```python
from build123d import *

# Parameters (mm, degrees)
SZKIC1_R                    = 40
DODANIE_WYCI_GNI_CIE1_DEPTH = 250
SZKIC2_W                    = 120
SZKIC2_H                    = 80
DODANIE_WYCI_GNI_CIE2_DEPTH = 10
SZKIC3_W                    = 10
SZKIC3_H                    = 80
DODANIE_WYCI_GNI_CIE3_DEPTH = 50


with BuildPart() as part:
    # Szkic1 → Dodanie-wyciągnięcie1 (new body)
    with BuildSketch(Plane.XY):
        Circle(SZKIC1_R)
    extrude(amount=DODANIE_WYCI_GNI_CIE1_DEPTH)

    # Szkic2 → Dodanie-wyciągnięcie2 (add)
    with BuildSketch(Plane.XY.offset(250)):
        Rectangle(SZKIC2_W, SZKIC2_H)
    extrude(amount=DODANIE_WYCI_GNI_CIE2_DEPTH)

    # Szkic3 → Dodanie-wyciągnięcie3 (add)
    with BuildSketch(Plane.XY.offset(260)):
        with Locations((-55, 0)):
            Rectangle(SZKIC3_W, SZKIC3_H)
        with Locations((55, 0)):
            Rectangle(SZKIC3_W, SZKIC3_H)
    extrude(amount=DODANIE_WYCI_GNI_CIE3_DEPTH)


solid = part.part
```
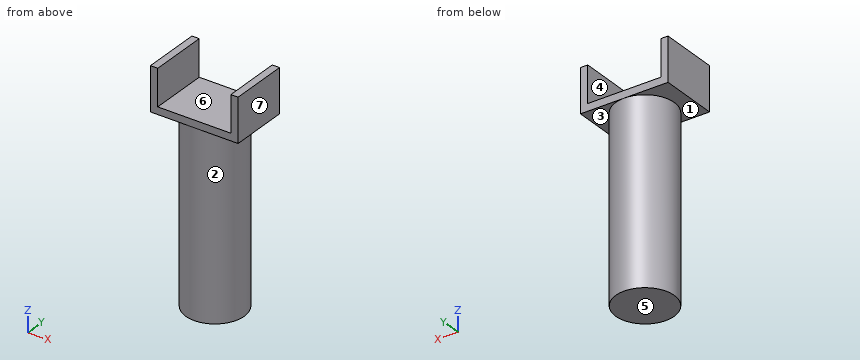
The model under review builds one solid part; all positions refer to its coordinate system, in mm. Face numbers are marked on the shaded views. A direction names the side the tool comes from. Round coordinates to 2 decimals unless told otherwise and drop trailing zeros. Loops run counter-clockwise (first coordinate to the right, second up) from the corner with the lowest first, then second, coordinate; pieces in that order, holes last. Notation, with made-up numbers: M 14.5,65.25 L 30.5,65.25 A12 cw 30.5,73.25 Z; hole C -3.75,48 d2. An arc over 180 degrees is marked long. Put each result on its own line as item: value.
Q1. Consider section C-C, the plane x = 34. Give the boundary of the cut face in (y, z).
Result set:
outline: M -40,250 L -21.07,250 L -21.07,0 L 21.07,0 L 21.07,250 L 40,250 L 40,260 L -40,260 Z
Q2. Consider section A-A, the plane z = 288.5. Give the boundary of the cut face in (x, y).
Result set:
outline: M -60,-40 L -50,-40 L -50,40 L -60,40 Z; M 50,-40 L 60,-40 L 60,40 L 50,40 Z
Q3. Consider section D-D, the plane z = 34. Give the boundary of the cut face in (x, y), then the cut area to 3 significant figures.
Result set:
outline: C 0,0 d80
area: 5,030 mm²
Q4. Consider section B-B, the plane y = 0. Give the boundary of the cut face in (x, z), then the cut area to 3 significant figures.
Result set:
outline: M -60,250 L -40,250 L -40,0 L 40,0 L 40,250 L 60,250 L 60,310 L 50,310 L 50,260 L -50,260 L -50,310 L -60,310 Z
area: 22,200 mm²
Q5. For pin 1 (4 mm diameter, centred on x = -6.5, z = 208.5, fed in from -Y); pin 2 (8 mm diameter, centred on y = 14.5, z = 73.5, fed in from -X); pin 3 (4 mm diameter, centred on x = 41.5, y = 10, fed in from -Z), all flat-tipped, find the tip position at first contact; note any pin that passes through.
Result set:
pin 1: stops at y = -39.75
pin 2: stops at x = -38.6
pin 3: stops at z = 250
Q6. To check wall thickness, follow L1, parallel to X at y = 20.5, z = 280.5; L2, parallel to Z at x = 23.5, y = 36; L3, parallel to Z at x = 23, y = 32. State the ranges of each line that lie inside material, in increasing order.
Result set:
L1: x = -60 to -50, 50 to 60
L2: z = 250 to 260
L3: z = 0 to 260
Q7. Machinability: for the marked faces 1, 2, 3 and 4, which of the approach directions +Z, -Z, +X, -X, +Y, -Y give a long, thin tool a straight path to every point of the face, cutting with its end or side? Answer none if there is none.
Result set:
face 1: -Z, -X
face 2: -Z
face 3: -Z, +X
face 4: +Z, +Y, -Y
Q8. Mouldability with a two-part tool opening along X and no side actions: class the marked faces 5, 6 and 7 as released by +X, released by -X, zero draft, split by the parting line, or undercut.
Result set:
face 5: zero draft
face 6: undercut
face 7: released by +X
